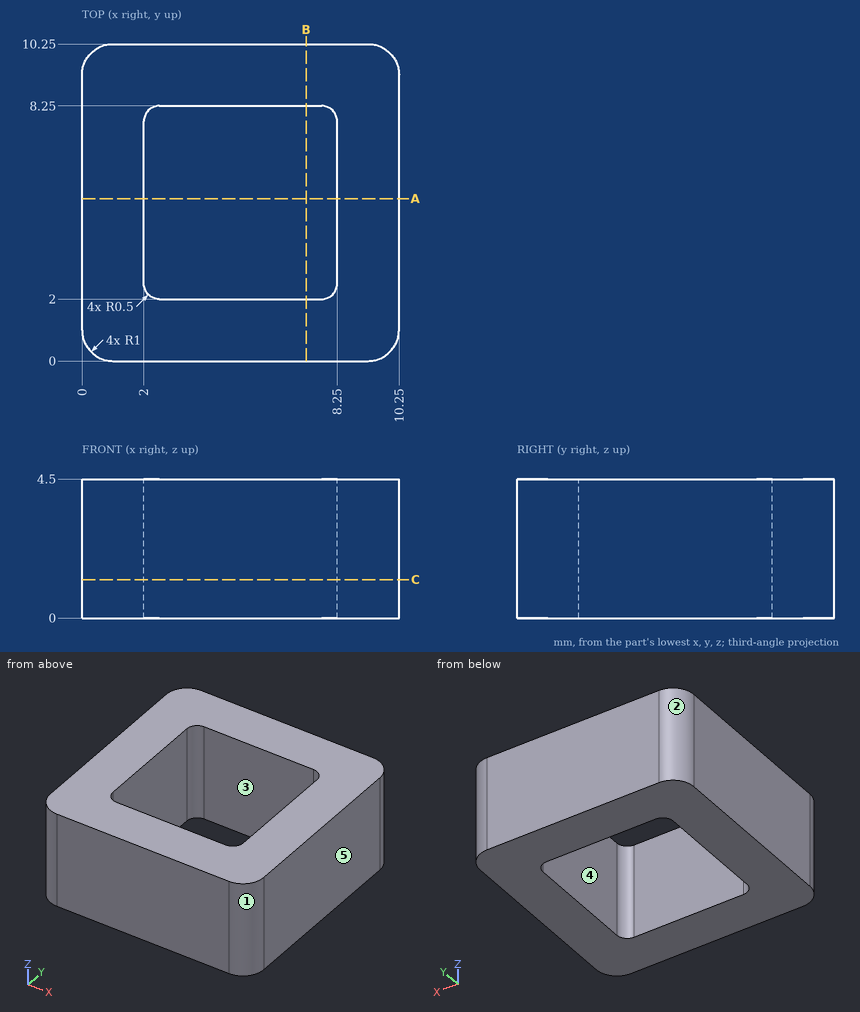
Could you check a few things on this drawing? It's one solid part, dimensions in mm from its lowest x, y, z. A direction names the side the tool comes from. Round coordinates to 2 decimals unless told otherwise and drop trailing zeros. Write each loop counter-clockwise with the first axis right and the second up, starting at its lowest first coordinate (ties: lowest second). Pieces come first, ordered by that corner, then holes. Notation, with made-up numbers: (2, -13) -> (19, -13) arc R22 ccw to (19, 22) -> close; hole circle Ø3 at (20.25, -18.75). An arc over 180 degrees is marked (long way). Use one line per item in the form item = value. Start each with the question number.
Q1. Imagine slicing it at C-C (z = 1.25). Please give me the cut outline in (x, y).
Q2. Imagine slicing it at A-A (y = 5.25). Please give me the cut outline in (x, z), then the cut area to 3 significant figures.
Q3. Which directions (+Z, -Z, +X, -X, +Y, -Y) give clear straight access to the entire face, cutting with the end or side of a thin tool? Please do the marked faces 4 and 5.
Q4. If I drill on probe 1 along X at (y, z) = (4.75, 2.7); probe 2 along X at (y, z) = (9.75, 2.45), over which ranges is the centre line in solid material (lowest first)? Write a range as [from, to].
Q5. We'd pull the mould along X, two halves only. Please class the marked faces 1, 2 and 3: +X half, -X half, draft (parallel to the pull), parting line (faces both ways), or undercut.
Worked out:
q1.outline = (0, 1) arc R1 ccw to (1, 0) -> (9.25, 0) arc R1 ccw to (10.25, 1) -> (10.25, 9.25) arc R1 ccw to (9.25, 10.25) -> (1, 10.25) arc R1 ccw to (0, 9.25) -> close; hole (2, 2.5) arc R0.5 ccw to (2.5, 2) -> (7.75, 2) arc R0.5 ccw to (8.25, 2.5) -> (8.25, 7.75) arc R0.5 ccw to (7.75, 8.25) -> (2.5, 8.25) arc R0.5 ccw to (2, 7.75) -> close
q2.outline = (0, 0) -> (2, 0) -> (2, 4.5) -> (0, 4.5) -> close; (8.25, 0) -> (10.25, 0) -> (10.25, 4.5) -> (8.25, 4.5) -> close
q2.area = 18.0 mm^2
q3.face_4 = +Z, -Z
q3.face_5 = +Z, -Z, +X, +Y, -Y
q4.probe_1 = [0, 2], [8.25, 10.25]
q4.probe_2 = [0.13, 10.12]
q5.face_1 = +X half
q5.face_2 = -X half
q5.face_3 = undercut
